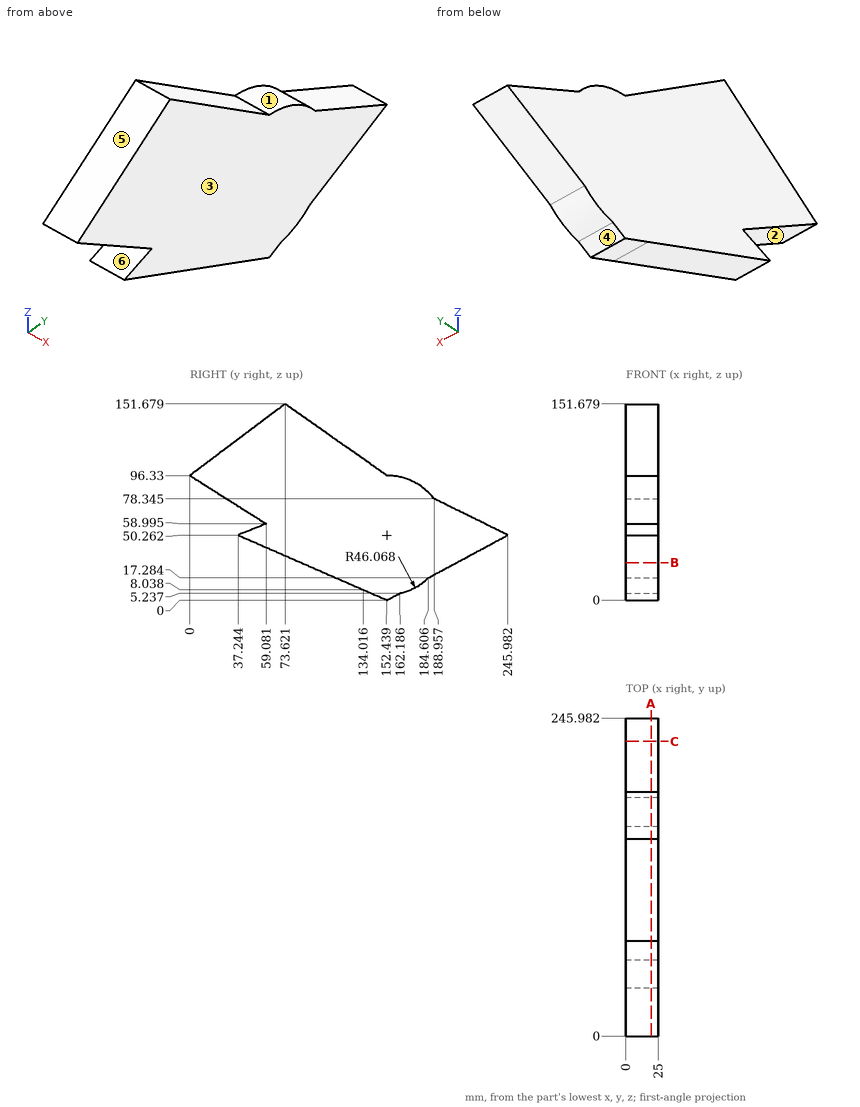
Job drawing, mm, ordinate dimensions from the low corner. One solid piece. A direction names the side the tool comes from. Coordinates: 2 decimals unless noted, no trailing zeros. Order: outer loops, then holes, each group sorted by start corner. A loop starts at its lowest first (then second) coordinate and runs counter-clockwise, first axis right, second up. Notation, with made-up numbers: (-12, 48) - (-2, 48) arc R18 ccw to (-2, 68) - close; hole circle Ø10 at (-12.5, -32.5). An arc over 180 degrees is marked (long way). Write each question's results on one line, items separated by ' | '. Start each with the question number.
Item 1: Band-saw the part on B-B on z = 29. Write the cut outline in (x, y) (1 decimal).
Item 2: Flat gauge pins, fed straight in: pin 1 (2 mm diameter, centred on x = 7.5, y = 98.5, fed in from +Z); pin 2 (2 mm diameter, centred on x = 11.5, y = 123, fed in from -Z); pin 3 (10 mm diameter, centred on x = 17, y = 161.5, fed in from +Z); pin 4 (12 mm diameter, centred on y = 31.5, z = 66, fed in from -X). Where does each tip first touch, or does it go through?
Item 3: Tool access for the marked faces 5 and 6: list every direction of +Z, -Z, +X, -X, +Y, -Y with a clear straight run to the whole face (end or side of a thin tool).
Item 4: Wall check: probe 1 along Z at (x, y) = (1.75, 53) (1 decimal); probe 2 along Z at (x, y) = (8, 50) (1 decimal); probe 3 along Y at (x, z) = (9.5, 139.5) (1 decimal). Give the ranges that are in metal, low to high. Write a range as [from, to].
Item 5: Band-saw the part on A-A on x = 19.5. Write the cut outline in (y, z) (1 decimal), and give its area (3 significant figures).
Item 6: Band-saw the part on C-C on y = 228. Write the cut outline in (x, z), and give its area (3 significant figures).
Item 7: Mould opens along Z. For the marked faces 1, 2, 3 and 4 say: released by +Z, released by -Z, zero draft, split by the parting line, or undercut.
Numbers:
1) outline: (0, 86) - (25, 86) - (25, 206.4) - (0, 206.4) - close
2) pin 1: z = 134.91 | pin 2: z = 12.41 | pin 3: z = 96.15 | pin 4: through
3) face 5: +Z, +X, -X, -Y | face 6: +X, -X, -Y
4) probe 1: [43.4, 56.6], [62.8, 136.2] | probe 2: [44.7, 55.4], [64.7, 133.9] | probe 3: [57.4, 91]
5) outline: (0, 96.3) - (59.1, 59) - (37.2, 50.3) - (152.4, 0) - (162.2, 5.2) arc R46.1 ccw to (184.6, 17.3) - (246, 50.3) - (189, 78.3) arc R46.1 ccw to (152.4, 96.3) - (73.6, 151.7) - close | area: 17,300 mm^2
6) outline: (0, 40.6) - (25, 40.6) - (25, 59.12) - (0, 59.12) - close | area: 463 mm^2
7) face 1: released by +Z | face 2: undercut | face 3: zero draft | face 4: released by -Z
